Verification items for this drawing (mm, ordinates from the low corner). A direction names the side the tool comes from. Coordinates: 2 decimals unless noted, no trailing zeros. Loops run counter-clockwise (first coordinate to the right, second up) from the corner with the lowest first, then second, coordinate; pieces in that order, holes last. Notation, with made-up numbers: (74, -23) -> (86, -23) arc R14 ccw to (86, -14) -> close; hole circle Ø9 at (66, -11.75). An arc over 180 degrees is marked (long way). Write item = value, one per line.
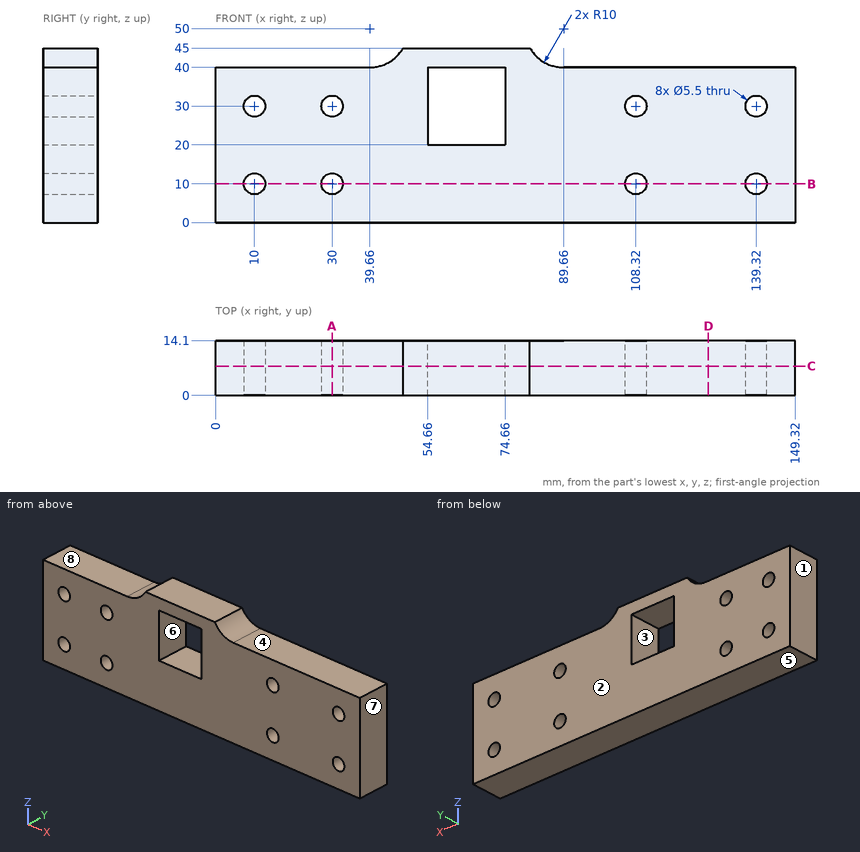
1) Sectioned sample at D-D, the plane x = 127. Record the cut outline in (y, z), plus the area to 3 significant figures.
Ans:
outline = (0, 0) -> (14.1, 0) -> (14.1, 40) -> (0, 40) -> close
area = 564 mm2
2) Tool access check on the marked faces 4, 5, 6, 7 and 8. Record the directions out of +Z, -Z, +X, -X, +Y, -Y that give a thin tool (end or side, any length) a straight path to the whole face; none if there is none.
Ans:
face_4 = +Z, +X, +Y, -Y
face_5 = -Z, +X, -X, +Y, -Y
face_6 = +Y, -Y
face_7 = +Z, -Z, +X, +Y, -Y
face_8 = +Z, -X, +Y, -Y
3) Sectioned sample at C-C, the plane y = 7.5. Count the separate pieces of the cut face and the enclosed holes in it, plus the area to 3 significant figures.
Ans:
separate_pieces = 1
enclosed_holes = 9
area = 5,570 mm2
4) Sectioned sample at B-B, the plane z = 10. Record the cut outline in (x, y), plus the area to 3 significant figures.
Ans:
outline = (0, 0) -> (7.25, 0) -> (7.25, 14.1) -> (0, 14.1) -> close; (12.75, 0) -> (27.25, 0) -> (27.25, 14.1) -> (12.75, 14.1) -> close; (32.75, 0) -> (105.57, 0) -> (105.57, 14.1) -> (32.75, 14.1) -> close; (111.07, 0) -> (136.57, 0) -> (136.57, 14.1) -> (111.07, 14.1) -> close; (142.07, 0) -> (149.32, 0) -> (149.32, 14.1) -> (142.07, 14.1) -> close
area = 1,800 mm2
5) Depth check by flat-ended pin: pin 1 Ø4.5 at (x, z) = (108.32, 30) entering from -Y. Enter the tip coordinate at first touch or a pass-through.
Ans:
pin_1 = through
6) Sectioned sample at A-A, the plane x = 30. Record the cut outline in (y, z), plus the area to 3 significant figures.
Ans:
outline = (0, 0) -> (14.1, 0) -> (14.1, 7.25) -> (0, 7.25) -> close; (0, 12.75) -> (14.1, 12.75) -> (14.1, 27.25) -> (0, 27.25) -> close; (0, 32.75) -> (14.1, 32.75) -> (14.1, 40) -> (0, 40) -> close
area = 409 mm2
7) Release check for a two-part mould opening along X. For the marked faces 1, 2 and 3 record: pulls with the +X half, pulls with the -X half, needs draft (parallel to the pull), parting line crosses it, or undercut.
Ans:
face_1 = pulls with the -X half
face_2 = needs draft
face_3 = undercut
8) Material ranges on line 1 (X direction, y = 5.5, z = 10); line 2 (X direction, y = 11, z = 30); line 3 (Z direction, x = 108.32, y = 3.5), recorded low to high.
Ans:
line_1 = 0 to 7.25, 12.75 to 27.25, 32.75 to 105.57, 111.07 to 136.57, 142.07 to 149.32
line_2 = 0 to 7.25, 12.75 to 27.25, 32.75 to 54.66, 74.66 to 105.57, 111.07 to 136.57, 142.07 to 149.32
line_3 = 0 to 7.25, 12.75 to 27.25, 32.75 to 40
